Geometry: final body of the model. Coordinates: model frame, mm. A direction names the side the tool comes from. Round coordinates to 2 decimals unless told otherwise and drop trailing zeros. Loops run counter-clockwise (first coordinate to the right, second up) from the corner with the lowest first, then second, coordinate; pieces in that order, holes last. Notation, with made-up numbers: M 79,35 L 104,35 A30 cw 104,74 Z; hole C -37.75,42.25 d10. An arc over 180 degrees is marked long. Answer as a JSON object with one key per item and string values.
from build123d import *

# Parameters (mm, degrees)
CUT_EXTRUDE2_DEPTH      = 90.451272324
CUT_EXTRUDE2_DEPTH_BACK = 90.451272324
SKETCH5_R               = 1.5
CUT_EXTRUDE3_START      = -2
SKETCH7_R               = 8
CUT_EXTRUDE3_DEPTH      = 2
BOSS_EXTRUDE1_START     = -2
SKETCH2_R               = 2.5
BOSS_EXTRUDE1_DEPTH     = 2


with BuildPart() as part:
    # Sketch1 → Revolve2 (revolve)
    with BuildSketch(Plane.XY, mode=Mode.PRIVATE) as revolve2_sk:
        Polygon((-85.136081821, -10.256002982), (-85.136081821, -18.256002982), (-75.136081821, -18.256002982), (-75.136081821, -10.256002982), (-77.136081821, -10.256002982), (-77.136081821, -12.256002982), (-83.136081821, -12.256002982), (-83.136081821, -10.256002982), align=None)
    revolve(revolve2_sk.sketch.rotate(Axis((-85.136081821, -18.256002982, 0), (1, 0, 0)), 90), axis=Axis((-85.136081821, -18.256002982, 0), (1, 0, 0)))

    # Sketch5 → Cut-Extrude2 (cut, two sides: drawn at the far end of the back side and taken through both)
    with BuildSketch(Plane.XY.offset(-CUT_EXTRUDE2_DEPTH_BACK)):
        with Locations((-80.136081821, -18.256002982)):
            Circle(SKETCH5_R)
    extrude(amount=CUT_EXTRUDE2_DEPTH + CUT_EXTRUDE2_DEPTH_BACK, mode=Mode.SUBTRACT)

    # Sketch7 → Cut-Extrude3 (cut)
    with BuildSketch(Plane(origin=(-75.136081821, 0, 0), x_dir=(0, 0, -1), z_dir=(1, 0, 0)).offset(CUT_EXTRUDE3_START)):
        with Locations(Location((0, -18.256002982, 0), (0, 0, 180))):
            Circle(SKETCH7_R)
    extrude(amount=CUT_EXTRUDE3_DEPTH, mode=Mode.SUBTRACT)

    # Sketch2 → Boss-Extrude1 (add)
    with BuildSketch(Plane(origin=(-75.136081821, 0, 0), x_dir=(0, 0, -1), z_dir=(1, 0, 0)).offset(BOSS_EXTRUDE1_START)):
        with Locations((0, -18.256002982)):
            Circle(SKETCH2_R)
    extrude(amount=BOSS_EXTRUDE1_DEPTH)


solid = part.part
1) Pin query (flat end, axial travel): P1, Ø6, axis at x = -80, z = 6, coming from the +Y side; P2, Ø1.5, axis at x = -81.5, z = 2.5, coming from the +Y side; P3, Ø1, axis at x = -79.5, y = -14, coming from the +Z side. Return the tip coordinate at first contact, or that it passes through.
Results:
{"P1": "y = -13.06", "P2": "y = -12.52", "P3": "z = 4.68"}
2) Reachability of faces 5 (the flat face through (-77.136, -18, 3)), 6 (the cylindrical face through (-84.2, -25, 4.3)) from +Z, -Z, +X, -X, +Y, -Y: full face, straight path, thin tool, end or side. Return the list, or none.
Results:
{"face 5": "+X", "face 6": "+X, -X"}
3) Section query A-A (z = -3). Return the cut outline in (x, y), and give its area (4 significant figures).
Results:
{"outline": "M -85.14,-25.67 L -83.14,-25.67 L -83.14,-23.45 L -77.14,-23.45 L -77.14,-13.06 L -83.14,-13.06 L -83.14,-10.84 L -85.14,-10.84 Z; hole C -80.14,-18.26 d3", "area": "84.95 mm2"}
4) Section query C-C (y = -13.75). Return the cut outline in (x, z), and give its area (3 significant figures).
Results:
{"outline": "M -85.14,-6.61 L -83.14,-6.61 L -83.14,-3.96 L -77.14,-3.96 L -77.14,3.96 L -83.14,3.96 L -83.14,6.61 L -85.14,6.61 Z", "area": "74.0 mm2"}
5) Section query D-D (x = -80). Return the cut outline in (y, z).
Results:
{"outline": "M -19.75,-5.81 L -19.75,5.81 A6 ccw Z; M -16.76,-5.81 A6 ccw -16.76,5.81 Z"}
6) Ray query, line 1 (Z direction, x = -78.25, y = -18.25); line 2 (X direction, y = -14.5, z = 3.5); line 3 (X direction, y = -12, z = -0.5). Return the intervals inside material, ascending.
Results:
{"line 1": "-6 to 6", "line 2": "-85.14 to -77.14", "line 3": "-85.14 to -83.14"}
7) Pull-direction query (X, two-part tool) for faces 1 (the cylindrical face through (-78.705, -17.805, -0.084)), 2 (the cylindrical face through (-76.15, -20.697, 0.542)), 3 (the flat face through (-75.136, -18, 0)), 4 (the flat face through (-85.136, -18, 0)); classes: +X half, -X half, draft (parallel to the pull), parting line (faces both ways), or undercut.
Results:
{"face 1": "undercut", "face 2": "draft", "face 3": "+X half", "face 4": "-X half"}
8) Section query B-B (y = -19.25). Return the cut outline in (x, z).
Results:
{"outline": "M -85.14,-7.94 L -83.14,-7.94 L -83.14,-5.92 L -81.26,-5.92 L -81.26,5.92 L -83.14,5.92 L -83.14,7.94 L -85.14,7.94 Z; M -79.01,-5.92 L -77.14,-5.92 L -77.14,-2.29 L -75.14,-2.29 L -75.14,2.29 L -77.14,2.29 L -77.14,5.92 L -79.01,5.92 Z"}
